For this review, take the finished solid that the model builds, in its own axes (mm). A direction names the side the tool comes from. Coordinates: 2 decimals unless noted, no trailing zeros. Write each loop counter-clockwise with the first axis right and the second up, starting at its lowest first coordinate (ties: lowest second). Pieces come first, ordered by that corner, then holes. Notation, with made-up numbers: (11.25, 51) - (54.25, 51) arc R27 ccw to (54.25, 78) - close; hole circle Ø7 at (5.25, 16.25). An arc over 180 degrees is marked (long way). Use one line per item in the form item = value. Start each with the question number.
1) We need section C-C (x = 2.5). Give the boundary of the cut face in (y, z).
2) We need section D-D (x = 25). Give the boundary of the cut face in (y, z), plus the area to 3 significant figures.
3) Tool access review of faces 1 (the conical face through (110.72, -1.22, -59.26)), 2 (the flat face through (35, -2, -2)): name each direction out of +Z, -Z, +X, -X, +Y, -Y from which nothing blocks a thin tool from reaching the whole face with its end or side.
4) Mouldability with a two-part tool opening along Z and no side actions: class faces 3 (the flat face through (8, -2, 0)), 4 (the flat face through (15, -2, -3)), 5 (the conical face through (4.43, -1.22, -60.08)) as pulls with the +Z half, pulls with the -Z half, needs draft (parallel to the pull), parting line crosses it, or undercut.
5) We need section B-B (z = -60). Give the boundary of the cut face in (x, y), plus the area to 3 significant figures.
6) Insertion check: P1, Ø4, axis at x = 112.5, z = -20, coming from the +Y side. The pin has a flat end and moves straight along its axis. Give the tip position at first contact, or say it passes through.
7) For L1, parallel to Z at x = 2.5, y = -3.15; L2, parallel to X at y = -4.3, z = -20; L3, parallel to X at y = -2.6, z = -19, list the stretches that pass through material, from the lowest coordinate up. Write a range as from..to.
8) We need section A-A (y = -3.75). Give the boundary of the cut face in (x, z), plus the area to 3 significant figures.
```python
from build123d import *

# Parameters (mm, degrees)
BOSS_EXTRUDE1_DEPTH                                 = 5
CSK_FOR_M3_FLAT_COUNTERSUNK_HEAD_SCREW1_D           = 3.4
CSK_FOR_M3_FLAT_COUNTERSUNK_HEAD_SCREW1_CSINK_D     = 6.3
CSK_FOR_M3_FLAT_COUNTERSUNK_HEAD_SCREW1_CSINK_ANGLE = 90


with BuildPart() as part:
    # Sketch1 → Boss-Extrude1 (new body)
    with BuildSketch(Plane(origin=(0, 0, 0), x_dir=(1, 0, 0), z_dir=(0, 1, 0))):
        with BuildLine():
            Line((15, 5), (15, 0))
            Line((15, 0), (0, 0))
            Line((0, 0), (0, 80))
            Line((0, 80), (115, 80))
            Line((115, 80), (115, 0))
            Line((115, 0), (35, 0))
            Line((35, 0), (35, 5))
            ThreePointArc((35, 5), (25, 15), (15, 5))
        make_face()
    extrude(amount=-BOSS_EXTRUDE1_DEPTH)

    # CSK for M3 Flat Countersunk Head Screw1 (through all)
    with Locations(Plane(origin=(0, 0, 0), x_dir=(1, 0, 0), z_dir=(0, 1, 0))):
        with Locations((2.5, 60), (2.5, 20), (112.5, 60), (112.5, 20)):
            CounterSinkHole(CSK_FOR_M3_FLAT_COUNTERSUNK_HEAD_SCREW1_D / 2, CSK_FOR_M3_FLAT_COUNTERSUNK_HEAD_SCREW1_CSINK_D / 2, counter_sink_angle=CSK_FOR_M3_FLAT_COUNTERSUNK_HEAD_SCREW1_CSINK_ANGLE)


solid = part.part
```
Determined:
q1.outline = (-5, -80) - (0, -80) - (0, -63.15) - (-1.45, -61.7) - (-5, -61.7) - close; (-5, -58.3) - (-1.45, -58.3) - (0, -56.85) - (0, -23.15) - (-1.45, -21.7) - (-5, -21.7) - close; (-5, -18.3) - (-1.45, -18.3) - (0, -16.85) - (0, 0) - (-5, 0) - close
q2.outline = (-5, -80) - (0, -80) - (0, -15) - (-5, -15) - close
q2.area = 325 mm²
q3.face_1 = +Y
q3.face_2 = +Z, +Y, -Y
q4.face_3 = pulls with the +Z half
q4.face_4 = needs draft
q4.face_5 = undercut
q5.outline = (0, -5) - (0.8, -5) - (0.8, -1.45) - (0, -0.65) - close; (4.2, -5) - (110.8, -5) - (110.8, -1.45) - (109.35, 0) - (5.65, 0) - (4.2, -1.45) - close; (114.2, -5) - (115, -5) - (115, -0.65) - (114.2, -1.45) - close
q5.area = 537 mm²
q6.P1 = -1.15
q7.L1 = -80..-61.7, -58.3..-21.7, -18.3..0
q7.L2 = 0..0.8, 4.2..110.8, 114.2..115
q7.L3 = 0..1.13, 3.87..111.13, 113.87..115
q8.outline = (0, -80) - (115, -80) - (115, 0) - (35, 0) - (35, -5) arc R10 cw to (15, -5) - (15, 0) - (0, 0) - close; hole circle Ø3.4 at (2.5, -60); hole circle Ø3.4 at (2.5, -20); hole circle Ø3.4 at (112.5, -60); hole circle Ø3.4 at (112.5, -20)
q8.area = 8,910 mm²
